from build123d import *

# Parameters (mm, degrees)
ESQUISSE1_W              = 32.25
ESQUISSE1_H              = 12.3
BOSS_EXTRU_1_DEPTH       = 5
ESQUISSE2_W              = 4.7
ESQUISSE2_H              = 12.3
BOSS_EXTRU_2_DEPTH       = 16.25
ESQUISSE5_W              = 32.25
ESQUISSE5_H              = 5
BOSS_EXTRU_4_DEPTH       = 27.9
ESQUISSE6_W              = 4.7
ESQUISSE6_H              = 3.8
BOSS_EXTRU_5_DEPTH       = 12.3
ESQUISSE7_W              = 32.25
ESQUISSE7_H              = 17.3
BOSS_EXTRU_6_DEPTH       = 4
ENL_V_MAT_EXTRU_2_DEPTH  = 4.3
ENL_V_START              = -12.3
ESQUISSE9_W              = 4.7
ESQUISSE9_H              = 1.6
ENL_V_MAT_EXTRU_3_DEPTH  = 12.3
ESQUISSE10_R             = 1
ENL_V_MAT_EXTRU_4_DEPTH  = 20.3
ESQUISSE16_W             = 32.25
ESQUISSE16_H             = 17.3
BOSS_EXTRU_8_DEPTH       = 14.1
ENL_V_START_2            = -17.3
ESQUISSE18_R             = 2
ENL_V_MAT_EXTRU_8_DEPTH  = 17.3
CONG_4_R                 = 6
ESQUISSE19_R             = 3.8
ENL_V_MAT_EXTRU_9_DEPTH  = 15.8
ESQUISSE20_W             = 4
ESQUISSE20_H             = 17.3
ENL_V_MAT_EXTRU_10_DEPTH = 2.5
ENL_V_MAT_EXTRU_11_DEPTH = 17.3
CONG_5_R                 = 6
CONG_6_R                 = 6
CONG_7_R                 = 1
CONG_8_R                 = 1
CONG_9_R                 = 0.5
CONG_10_R                = 0.5
CONG_11_R                = 0.5


with BuildPart() as part:
    # Esquisse1 → Boss.-Extru.1 (new body)
    with BuildSketch(Plane.XY):
        with Locations((16.125, -6.15)):
            Rectangle(ESQUISSE1_W, ESQUISSE1_H)
    extrude(amount=BOSS_EXTRU_1_DEPTH)

    # Esquisse2 → Boss.-Extru.2 (add)
    with BuildSketch(Plane.XY.offset(5)):
        with Locations((2.35, -6.15)):
            Rectangle(ESQUISSE2_W, ESQUISSE2_H)
        with Locations((29.9, -6.15)):
            Rectangle(ESQUISSE2_W, ESQUISSE2_H)
    extrude(amount=BOSS_EXTRU_2_DEPTH)

    # Esquisse5 → Boss.-Extru.4 (add)
    with BuildSketch(Plane(origin=(0, 0, 0), x_dir=(-1, 0, 0), z_dir=(0, 0, -1))):
        with Locations((-16.125, 2.5)):
            Rectangle(ESQUISSE5_W, ESQUISSE5_H)
    extrude(amount=-BOSS_EXTRU_4_DEPTH)

    # Esquisse6 → Boss.-Extru.5 (add)
    with BuildSketch(Plane.XZ):
        with Locations((29.9, 26)):
            Rectangle(ESQUISSE6_W, ESQUISSE6_H)
        with Locations((2.35, 26)):
            Rectangle(ESQUISSE6_W, ESQUISSE6_H)
    extrude(amount=BOSS_EXTRU_5_DEPTH)

    # Esquisse7 → Boss.-Extru.6 (add)
    with BuildSketch(Plane.XY.offset(27.9)):
        with Locations((16.125, -3.65)):
            Rectangle(ESQUISSE7_W, ESQUISSE7_H)
    extrude(amount=BOSS_EXTRU_6_DEPTH)

    # Esquisse8 → Enlèv. mat.-Extru.2 (cut)
    with BuildSketch(Plane.XY.offset(31.9)):
        with BuildLine():
            Line((12.62, -5.85), (12.62, -12.3))
            Line((12.62, -12.3), (27.27, -12.3))
            Line((27.27, -12.3), (27.27, -5.85))
            ThreePointArc((27.27, -5.85), (22.934690305, -0.315777347), (16.523466536, -3.2))
            Line((16.523466536, -3.2), (15.27, -3.2))
            ThreePointArc((15.27, -3.2), (13.39616703, -3.97616703), (12.62, -5.85))
        make_face()
    extrude(amount=-ENL_V_MAT_EXTRU_2_DEPTH, mode=Mode.SUBTRACT)

    # Esquisse9 → Enlèv. mat.-Extru.3 (cut)
    with BuildSketch(Plane.XZ.offset(12.3).offset(ENL_V_START)):
        with Locations((29.9, 10.8)):
            Rectangle(ESQUISSE9_W, ESQUISSE9_H)
    extrude(amount=ENL_V_MAT_EXTRU_3_DEPTH, mode=Mode.SUBTRACT)

    # Esquisse10 → Enlèv. mat.-Extru.4 (cut)
    with BuildSketch(Plane.XY.offset(31.9)):
        with Locations((30.25, -6.15)):
            Circle(ESQUISSE10_R)
        with Locations((2, -6.15)):
            Circle(ESQUISSE10_R)
    extrude(amount=-ENL_V_MAT_EXTRU_4_DEPTH, mode=Mode.SUBTRACT)

    # Esquisse16 → Boss.-Extru.8 (add)
    with BuildSketch(Plane(origin=(0, 0, 0), x_dir=(-1, 0, 0), z_dir=(0, 0, -1))):
        with Locations((-16.125, -3.65)):
            Rectangle(ESQUISSE16_W, ESQUISSE16_H)
    extrude(amount=BOSS_EXTRU_8_DEPTH)

    # Esquisse18 → Enlèv. mat.-Extru.8 (cut)
    with BuildSketch(Plane(origin=(0, 5, 0), x_dir=(1, 0, 0), z_dir=(0, 1, 0)).offset(ENL_V_START_2)):
        with Locations(Location((15.25, -24.1, 0), (0, 0, 270))):
            Circle(ESQUISSE18_R)
        with Locations(Location((15.25, 5.9, 0), (0, 0, 270))):
            Circle(ESQUISSE18_R)
    extrude(amount=ENL_V_MAT_EXTRU_8_DEPTH, mode=Mode.SUBTRACT)

    # Congé4
    cong_4_edges = [part.edges().sort_by_distance(p)[0] for p in [
        (0, -3.65, -14.1),
    ]]
    fillet(cong_4_edges, radius=CONG_4_R)

    # Esquisse19 → Enlèv. mat.-Extru.9 (cut)
    with BuildSketch(Plane.XZ.offset(12.3)):
        with Locations(Location((15.25, -5.9, 0), (0, 0, 270))):
            Circle(ESQUISSE19_R)
        with Locations(Location((15.25, 24.1, 0), (0, 0, 270))):
            Circle(ESQUISSE19_R)
    extrude(amount=-ENL_V_MAT_EXTRU_9_DEPTH, mode=Mode.SUBTRACT)

    # Esquisse20 → Enlèv. mat.-Extru.10 (cut)
    with BuildSketch(Plane.XY.offset(31.9)):
        with Locations((2, -3.65)):
            Rectangle(ESQUISSE20_W, ESQUISSE20_H)
        with Locations((30.25, -3.65)):
            Rectangle(ESQUISSE20_W, ESQUISSE20_H)
    extrude(amount=-ENL_V_MAT_EXTRU_10_DEPTH, mode=Mode.SUBTRACT)

    # Esquisse22 → Enlèv. mat.-Extru.11 (cut)
    with BuildSketch(Plane.XZ.offset(12.3).offset(ENL_V_START_2)):
        Polygon((19.038139385, -14.1), (32.25, -2.1), (32.25, -14.1), align=None)
    extrude(amount=ENL_V_MAT_EXTRU_11_DEPTH, mode=Mode.SUBTRACT)

    # Congé5
    cong_5_edges = [part.edges().sort_by_distance(p)[0] for p in [
        (19.038139385, -3.65, -14.1),
    ]]
    fillet(cong_5_edges, radius=CONG_5_R)

    # Congé6
    cong_6_edges = [part.edges().sort_by_distance(p)[0] for p in [
        (32.25, -3.65, -2.1),
    ]]
    fillet(cong_6_edges, radius=CONG_6_R)

    # Congé7
    cong_7_edges = [part.edges().sort_by_distance(p)[0] for p in [
        (32.25, -3.65, 29.4),
    ]]
    fillet(cong_7_edges, radius=CONG_7_R - 0.0001)  # a hair under: the kernel refuses the full size

    # Congé8
    cong_8_edges = [part.edges().sort_by_distance(p)[0] for p in [
        (0, -3.65, 29.4),
    ]]
    fillet(cong_8_edges, radius=CONG_8_R - 0.0001)  # a hair under: the kernel refuses the full size

    # Congé9
    cong_9_edges = [part.edges().sort_by_distance(p)[0] for p in [
        (28.25, -3.65, 31.9),
    ]]
    fillet(cong_9_edges, radius=CONG_9_R)

    # Congé10
    cong_10_edges = [part.edges().sort_by_distance(p)[0] for p in [
        (4, -3.65, 31.9),
    ]]
    fillet(cong_10_edges, radius=CONG_10_R)

    # Congé11
    cong_11_edges = [part.edges().sort_by_distance(p)[0] for p in [
        (27.55, -6.15, 10),
        (27.55, -6.15, 11.6),
        (4.7, -6.15, 21.25),
        (27.55, -6.15, 21.25),
        (27.55, -6.15, 24.1),
        (4.7, -6.15, 24.1),
    ]]
    fillet(cong_11_edges, radius=CONG_11_R)


solid = part.part
Geometry: final body of the model. Coordinates: model frame, mm. A direction names the side the tool comes from. Round coordinates to 2 decimals unless told otherwise and drop trailing zeros. Loops run counter-clockwise (first coordinate to the right, second up) from the corner with the lowest first, then second, coordinate; pieces in that order, holes last.
Q1. Section D-D on x = 2. Return loops of the section in (y, z), plus the area to 3 significant figures.
Q2. Section C-C on y = -10.75. State how many separate pieces and enclosed holes the cut face has, plus the area to 3 significant figures.
Q3. Access query for faces 4 (the cylindrical face through (23.037, -0.342, 29.928)), 5 (the flat face through (28.25, -4, 30)), 6 (the cylindrical face through (29.513, -5.474, 16.493)), 7 (the flat face through (2, -4, 29.4)). Directions: +Z, -Z, +X, -X, +Y, -Y. A direction counts if a zero-diameter tool reaches every point of the face in a straight line with its end or side. Return the directions, or none.
Q4. Section B-B on z = 14. Return loops of the section in (x, y).
Q5. Pin query (flat end, axial travel): P1, Ø4.5, axis at x = 15.25, z = 24.1, coming from the -Y side; P2, Ø2.5, axis at x = 30.25, y = -6.15, coming from the +Z side; P3, Ø4, axis at y = -1.5, z = -5.5, coming from the +X side. Return the tip coordinate at first contact, or that it passes through.
Q6. Material intervals for L1, parallel to Z at x = 14, y = 2.25; L2, parallel to X at y = -4.75, z = 14; L3, parallel to Z at x = 9.5, y = -6, sorted ascending.
Q7. Pull-direction query (Y, two-part tool) for faces 1 (the flat face through (2, -6, 11.6)), 2 (the flat face through (27.55, -6, 26)), 3 (the flat face through (13, -12.3, 0)); classes: released by +Y, released by -Y, zero draft, split by the parting line, or undercut.
Q8. Section A-A on y = 2. Return loops of the section in (x, z).
Evaluation:
1. outline: (-12.3, -12.57) - (5, -12.57) - (5, 29.4) - (-5.15, 29.4) - (-5.15, 24.1) - (0, 24.1) - (0, 21.25) - (-5.15, 21.25) - (-5.15, 11.6) - (-7.15, 11.6) - (-7.15, 21.25) - (-12.3, 21.25) - close; (-12.3, 24.1) - (-7.15, 24.1) - (-7.15, 29.4) - (-12.3, 29.4) - close
1. area: 661 mm2
2. separate pieces: 4
2. enclosed holes: 1
2. area: 713 mm2
3. face 4: +Z, -Y
3. face 5: +Z, +X, +Y, -Y
3. face 6: +Z
3. face 7: +Z, -X, +Y, -Y
4. outline: (0, -12.3) - (4.7, -12.3) - (4.7, 0) - (27.55, 0) - (27.55, -12.3) - (32.25, -12.3) - (32.25, 5) - (0, 5) - close; hole circle Ø2 at (2, -6.15); hole circle Ø2 at (30.25, -6.15)
5. P1: stops at y = 3.5
5. P2: stops at z = 29.4
5. P3: stops at x = 30.67
6. L1: z = -14.1 to -9.49, -2.31 to 20.51, 27.69 to 31.9
6. L2: x = 0 to 4.7, 27.55 to 32.25
6. L3: z = -14.1 to 5, 27.9 to 31.9
7. face 1: undercut
7. face 2: zero draft
7. face 3: released by -Y
8. outline: (0, -8.1) arc R6 ccw to (6, -14.1) - (16.72, -14.1) arc R6 ccw to (20.75, -12.54) - (30.28, -3.89) arc R6 ccw to (32.25, 0.56) - (32.25, 28.4) arc R1 ccw to (31.25, 29.4) - (28.25, 29.4) - (28.25, 31.4) arc R0.5 ccw to (27.75, 31.9) - (4.5, 31.9) arc R0.5 ccw to (4, 31.4) - (4, 29.4) - (1, 29.4) arc R1 ccw to (0, 28.4) - close; hole circle Ø7.6 at (15.25, -5.9); hole circle Ø7.6 at (15.25, 24.1)
